Answer from the drawing. Dimensions are ordinates in mm from the lowest x, y and z of the part. A direction names the side the tool comes from. Round coordinates to 2 decimals unless told otherwise and drop trailing zeros. Write each loop counter-clockwise with the first axis right and the second up, starting at its lowest first coordinate (ties: lowest second). Pieces come first, ordered by that corner, then holes.
1. Find section D-D (x = 4.5). Write down the section's boundary in (y, z).
2. Flat-ended cylindrical pins translate along their axes: pin 1 Ø3 at (x, z) = (5.5, 13) entering from -Y; pin 2 Ø2 at (x, z) = (3.5, 5.5) entering from +Y; pin 3 Ø1.1 at (y, z) = (6.5, 6.5) entering from +X. Find the tip coordinate at first contact, or state that the pin passes through.
3. Find section A-A (x = 6.5). Write down the section's boundary in (y, z), and give its area (3 significant figures).
4. A tool of negligible diameter and unlimited length cuts with its end or side. For the marked faces 1, 2 and 3, from which of +Z, -Z, +X, -X, +Y, -Y can it reach the whole face along a straight path? Write none if from no direction.
5. Find section C-C (y = 6.5). Write down the section's boundary in (x, z), and give its area (3 significant figures).
6. Find section B-B (z = 13). Write down the section's boundary in (x, y).
7. Straight lines are drawn through the part: probe 1 along Z at (x, y) = (6.5, 6.7); probe 2 along X at (y, z) = (6.35, 13); probe 3 along Z at (x, y) = (0.75, 5.25). For each, find the intervals that lie inside material, in ascending order.
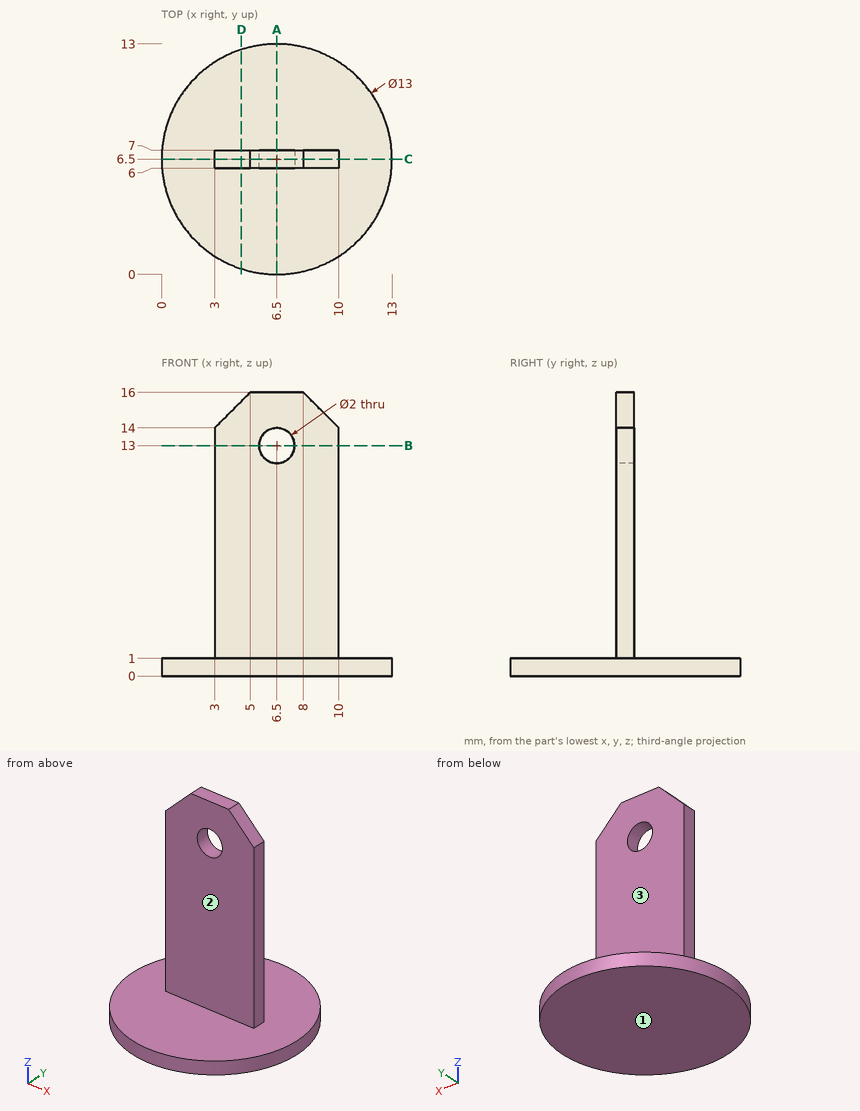
Worked answers:
1. outline: (0.32, 0) - (12.68, 0) - (12.68, 1) - (7, 1) - (7, 15.5) - (6, 15.5) - (6, 1) - (0.32, 1) - close
2. pin 1: stops at y = 6
2. pin 2: stops at y = 7
2. pin 3: stops at x = 10
3. outline: (0, 0) - (13, 0) - (13, 1) - (7, 1) - (7, 12) - (6, 12) - (6, 1) - (0, 1) - close; (6, 14) - (7, 14) - (7, 16) - (6, 16) - close
3. area: 26.0 mm2
4. face 1: -Z, +X, -X, +Y, -Y
4. face 2: +Z, +X, -X, -Y
4. face 3: +Z, +X, -X, +Y
5. outline: (0, 0) - (13, 0) - (13, 1) - (10, 1) - (10, 14) - (8, 16) - (5, 16) - (3, 14) - (3, 1) - (0, 1) - close; hole circle Ø2 at (6.5, 13)
5. area: 111 mm2
6. outline: (3, 6) - (5.5, 6) - (5.5, 7) - (3, 7) - close; (7.5, 6) - (10, 6) - (10, 7) - (7.5, 7) - close
7. probe 1: z = 0 to 12, 14 to 16
7. probe 2: x = 3 to 5.5, 7.5 to 10
7. probe 3: z = 0 to 1
